```python
from build123d import *

# Parameters (mm, degrees)
F0_R     = 12.7
F1_DEPTH = 6.35


# Not quite as in the source:
# - a length typed as a fraction of an inch, garbled in the dataset ("3 / 203.2 mm" for 3/8 in), is restored


with BuildPart() as f1:
    # F0 (on Top) → F1 (new body)
    with BuildSketch(Plane.XY):
        with BuildLine():
            ThreePointArc((-73.6864583333, -31.6503492602), (-59.3280711503, -33.8428959089), (-47.4486111111, -42.2004656802))
            ThreePointArc((-47.4486111111, -42.2004656802), (0, -63.5), (47.4486111111, -42.2004656802))
            ThreePointArc((47.4486111111, -42.2004656802), (59.3280711503, -33.8428959089), (73.6864583333, -31.6503492602))
            ThreePointArc((73.6864583333, -31.6503492602), (107.95, 0), (73.6864583333, 31.6503492602))
            ThreePointArc((73.6864583333, 31.6503492602), (59.3280711503, 33.8428959089), (47.4486111111, 42.2004656802))
            ThreePointArc((47.4486111111, 42.2004656802), (0, 63.5), (-47.4486111111, 42.2004656802))
            ThreePointArc((-47.4486111111, 42.2004656802), (-59.3280711503, 33.8428959089), (-73.6864583333, 31.6503492602))
            ThreePointArc((-73.6864583333, 31.6503492602), (-107.95, 0), (-73.6864583333, -31.6503492602))
        make_face()
        with Locations((-76.2, 0)):
            Circle(F0_R, mode=Mode.SUBTRACT)
        with BuildLine():
            ThreePointArc((0, 44.45), (31.4308964237, 31.4308964237), (44.45, 0))
            ThreePointArc((44.45, 0), (31.4308964237, -31.4308964237), (0, -44.45))
            ThreePointArc((0, -44.45), (-44.45, 0), (0, 44.45))
        make_face(mode=Mode.SUBTRACT)
        with Locations((76.2, 0)):
            Circle(F0_R, mode=Mode.SUBTRACT)
    extrude(amount=F1_DEPTH)


solid = f1.part
```
The model under review builds one solid part; all positions refer to its coordinate system, in mm. Coordinates: 2 decimals unless noted, no trailing zeros. Order: outer loops, then holes, each group sorted by start corner. A loop starts at its lowest first (then second) coordinate and runs counter-clockwise, first axis right, second up. Notation, with made-up numbers: (-22, 57.5) -> (26, 57.5) arc R22 cw to (26, 88.5) -> close; hole circle Ø10 at (11, 52). An arc over 180 degrees is marked (long way). Answer in a Markdown table with one row per item. Add a question column.
Item 1: We need section A-A on x = 76.2. Write out the cut boundary in (y, z).
Item 2: Mouldability with a two-part tool opening along X and no side actions: class faces 1 (the flat face through (46, 1, 6.35)), 2 (the cylindrical face through (63.512, 0.558, 3.131)), 3 (the cylindrical face through (-0.75, -63.496, 3.131)) as +X half, -X half, draft (parallel to the pull), parting line (faces both ways), or undercut.
Item 3: We need section D-D on z = 1. Write out the cut boundary in (x, y), plus the area to 3 significant figures.
Item 4: Clearance check with flat-ended pins moving along their axes: pin 1 (3 mm diameter, centred on y = -24, z = 3, fed in from +X); pin 2 (2 mm diameter, centred on y = 16, z = 5, fed in from +X); pin 3 (1.5 mm diameter, centred on y = 1.5, z = 4, fed in from -X). State where each tip first meets the part, or that it passes through.
Item 5: We need section C-C on y = -27. Write out the cut boundary in (x, z), plus the area to 3 significant figures.
Item 6: To check wall thickness, follow probe 1 along Y at (x, z) = (76.2, 4.75); probe 2 along X at (y, z) = (38.5, 4); probe 3 along Y at (x, z) = (13, 3). State the ranges of each line that lie inside material, in increasing order.
Item 7: We need section B-B on y = 10. Write out the cut boundary in (x, z), plus the area to 3 significant figures.
Final values:
| question | item | result |
|---|---|---|
| 1 | outline | (-31.75, 0) -> (-12.7, 0) -> (-12.7, 6.35) -> (-31.75, 6.35) -> close; (12.7, 0) -> (31.75, 0) -> (31.75, 6.35) -> (12.7, 6.35) -> close |
| 2 | face 1 | draft |
| 2 | face 2 | undercut |
| 2 | face 3 | parting line |
| 3 | outline | (-73.69, -31.65) arc R31.75 cw to (-47.45, -42.2) arc R63.5 ccw to (47.45, -42.2) arc R31.75 cw to (73.69, -31.65) arc R31.75 ccw (long way) to (73.69, 31.65) arc R31.75 cw to (47.45, 42.2) arc R63.5 ccw to (-47.45, 42.2) arc R31.75 cw to (-73.69, 31.65) arc R31.75 ccw (long way) to start; hole circle Ø25.4 at (-76.2, 0); hole circle Ø88.9 at (0, 0); hole circle Ø25.4 at (76.2, 0) |
| 3 | area | 10,700 mm2 |
| 4 | pin 1 | stops at x = 98.6 |
| 4 | pin 2 | stops at x = 104.18 |
| 4 | pin 3 | stops at x = -107.94 |
| 5 | outline | (-92.91, 0) -> (-35.31, 0) -> (-35.31, 6.35) -> (-92.91, 6.35) -> close; (35.31, 0) -> (92.91, 0) -> (92.91, 6.35) -> (35.31, 6.35) -> close |
| 5 | area | 731 mm2 |
| 6 | probe 1 | y = -31.75 to -12.7, 12.7 to 31.75 |
| 6 | probe 2 | x = -51.35 to -22.22, 22.22 to 51.35 |
| 6 | probe 3 | y = -62.16 to -42.51, 42.51 to 62.16 |
| 7 | outline | (-106.33, 0) -> (-84.03, 0) -> (-84.03, 6.35) -> (-106.33, 6.35) -> close; (-68.37, 0) -> (-43.31, 0) -> (-43.31, 6.35) -> (-68.37, 6.35) -> close; (43.31, 0) -> (68.37, 0) -> (68.37, 6.35) -> (43.31, 6.35) -> close; (84.03, 0) -> (106.33, 0) -> (106.33, 6.35) -> (84.03, 6.35) -> close |
| 7 | area | 602 mm2 |
